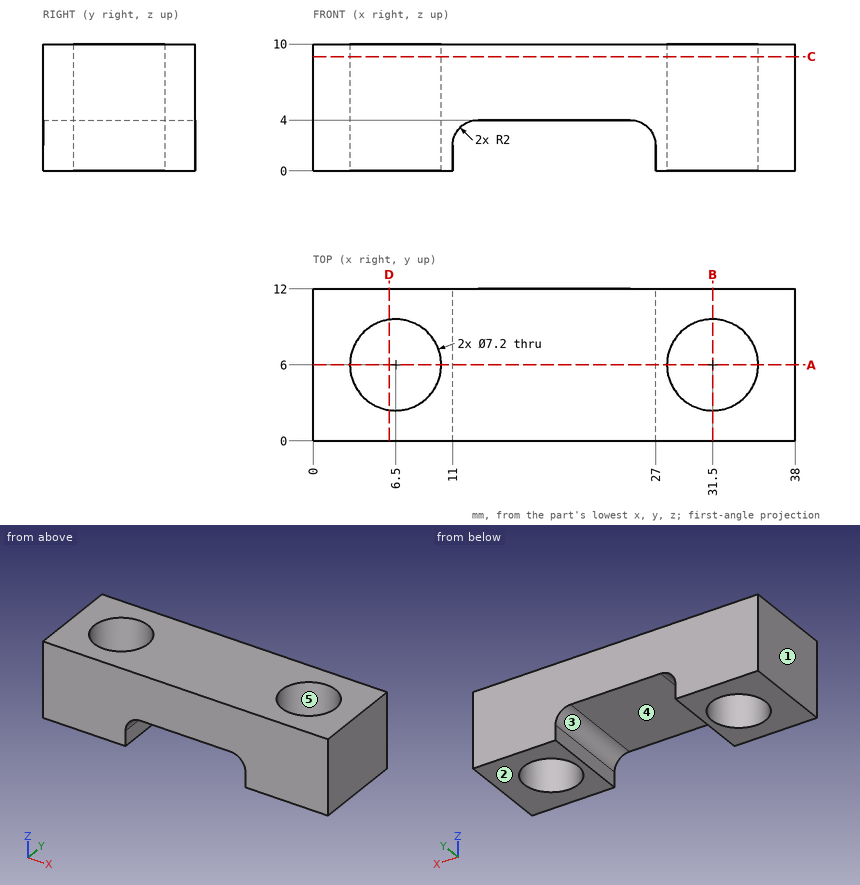
Verification items for this drawing (mm, ordinates from the low corner). A direction names the side the tool comes from. Give positions to 0.01 mm unless a question says otherwise; leave off trailing zeros. Write each loop counter-clockwise with the first axis right and the second up, starting at its lowest first coordinate (ties: lowest second). Pieces come first, ordered by that corner, then holes. Notation, with made-up numbers: (9, 73) - (42, 73) arc R19 ccw to (42, 77) - close; hole circle Ø3 at (-13.75, 58.25). An arc over 180 degrees is marked (long way). Answer as CSV lines item,"result". Start each with the question number.
1. Sectioned sample at B-B (x = 31.5). Record the boundary of the cut face in (y, z), then the cut area to 3 significant figures.
2. Set-up check for the marked faces 4 and 5: record each of +Z, -Z, +X, -X, +Y, -Y from which the full face is reachable in a straight line by a thin tool's end or side.
3. Depth check by flat-ended pin: pin 1 (1.5 mm diameter, centred on x = 17, y = 7.5, fed in from -Z); pin 2 (3 mm diameter, centred on x = 19, z = 2, fed in from +Y). Enter the tip coordinate at first touch or a pass-through.
4. Sectioned sample at D-D (x = 6). Record the boundary of the cut face in (y, z), then the cut area to 3 significant figures.
5. Draft check along X on the marked faces 1, 2 and 3. Enter one of: pulls with the +X half, pulls with the -X half, needs draft (parallel to the pull), parting line crosses it, or undercut.
6. Thickness scan on line 1 (Y direction, x = 6.5, z = 2.25); line 2 (X direction, y = 4.5, z = 7.75); line 3 (X direction, y = 3.25, z = 3). Record the ranges inside material, lowest first.
7. Sectioned sample at C-C (z = 9). Record the boundary of the cut face in (x, y).
8. Sectioned sample at A-A (y = 6). Record the boundary of the cut face in (x, z), then the cut area to 3 significant figures.
Derived:
1,outline,"(0, 0) - (2.4, 0) - (2.4, 10) - (0, 10) - close; (9.6, 0) - (12, 0) - (12, 10) - (9.6, 10) - close"
1,area,"48.0 mm²"
2,face 4,"-Z, +Y, -Y"
2,face 5,"+Z, -Z"
3,pin 1,"z = 4"
3,pin 2,"through"
4,outline,"(0, 0) - (2.43, 0) - (2.43, 10) - (0, 10) - close; (9.57, 0) - (12, 0) - (12, 10) - (9.57, 10) - close"
4,area,"48.7 mm²"
5,face 1,"pulls with the -X half"
5,face 2,"needs draft"
5,face 3,"undercut"
6,line 1,"0 to 2.4, 9.6 to 12"
6,line 2,"0 to 3.23, 9.77 to 28.23, 34.77 to 38"
6,line 3,"0 to 4.18, 8.82 to 11.27, 26.73 to 29.18, 33.82 to 38"
7,outline,"(0, 0) - (38, 0) - (38, 12) - (0, 12) - close; hole circle Ø7.2 at (6.5, 6); hole circle Ø7.2 at (31.5, 6)"
8,outline,"(0, 0) - (2.9, 0) - (2.9, 10) - (0, 10) - close; (10.1, 0) - (11, 0) - (11, 2) arc R2 cw to (13, 4) - (25, 4) arc R2 cw to (27, 2) - (27, 0) - (27.9, 0) - (27.9, 10) - (10.1, 10) - close; (35.1, 0) - (38, 0) - (38, 10) - (35.1, 10) - close"
8,area,"174 mm²"
